CAD build for the part. Positions are in the model's coordinates, mm. A direction names the side the tool comes from. Give positions to 0.01 mm unless a question says otherwise; leave off trailing zeros. Loops run counter-clockwise (first coordinate to the right, second up) from the corner with the lowest first, then second, coordinate; pieces in that order, holes last. Notation, with made-up numbers: (25, 30) -> (59, 30) arc R15 ccw to (59, 42) -> close; hole circle Ø7 at (56, 12.5). An arc over 180 degrees is marked (long way). Write each question's results on one line, items separated by ' | '. Start each with the question number.
```python
from build123d import *

# Parameters (mm, degrees)
F0_R     = 50.8
F1_DEPTH = 10.16
F2_R     = 48.4632
F3_DEPTH = 10.16
F4_R     = 43.9928
F5_DEPTH = 10.16
F6_R     = 36.2712
F7_DEPTH = 10.16
F8_R     = 22.1488
F9_DEPTH = 10.16


with BuildPart() as f1:
    # F0 (on Top) → F1 (new body)
    with BuildSketch(Plane.XY):
        Circle(F0_R)
    extrude(amount=F1_DEPTH)

    # F2 (on face) → F3 (join)
    with BuildSketch(Plane.XY.offset(10.16)):
        Circle(F2_R)
    extrude(amount=F3_DEPTH)

    # F4 (on face) → F5 (join)
    with BuildSketch(Plane.XY.offset(20.32)):
        Circle(F4_R)
    extrude(amount=F5_DEPTH)

    # F6 (on face) → F7 (join)
    with BuildSketch(Plane.XY.offset(30.48)):
        Circle(F6_R)
    extrude(amount=F7_DEPTH)

    # F8 (on face) → F9 (join)
    with BuildSketch(Plane.XY.offset(40.64)):
        Circle(F8_R)
    extrude(amount=F9_DEPTH)


solid = f1.part
```
Q1. Which spindle directions (+Z, -Z, +X, -X, +Y, -Y) get a long thin tool onto all of the face, cutting with end or side? Do faces 1 (the face through (-34.91, -26.77, 25.33)), 2 (the face through (0, 0, 50.8)). Say none if no direction does.
Q2. Drop flat-ended pins along their axis: pin 1 (4 mm diameter, centred on x = -4.5, z = 10.5, fed in from -Y); pin 2 (4 mm diameter, centred on x = -20, y = 25.5, fed in from +Z); pin 3 (1 mm diameter, centred on y = -2, z = 13, fed in from +X). Give the stop position or say it passes through.
Q3. Saw through at A-A, the plane x = 0. List the corners of the cut face in (y, z), then the cut area to 3 significant figures.
Q4. Wall check: L1, parallel to Z at x = 2, y = 36; L2, parallel to Z at x = -22.5, y = -39; L3, parallel to X at y = 6, z = 4.5. Give the ranges that are in metal, low to high.
Q5. Saw through at D-D, the plane x = -25. List the corners of the cut face in (y, z), then the cut area to 3 significant figures.
Q6. Saw through at C-C, the plane z = 15. List the corners of the cut face in (x, y).
Answer block:
1) face 1: +Z | face 2: +Z, +X, -X, +Y, -Y
2) pin 1: stops at y = -50.74 | pin 2: stops at z = 40.64 | pin 3: stops at x = 48.44
3) outline: (-50.8, 0) -> (50.8, 0) -> (50.8, 10.16) -> (48.46, 10.16) -> (48.46, 20.32) -> (43.99, 20.32) -> (43.99, 30.48) -> (36.27, 30.48) -> (36.27, 40.64) -> (22.15, 40.64) -> (22.15, 50.8) -> (-22.15, 50.8) -> (-22.15, 40.64) -> (-36.27, 40.64) -> (-36.27, 30.48) -> (-43.99, 30.48) -> (-43.99, 20.32) -> (-48.46, 20.32) -> (-48.46, 10.16) -> (-50.8, 10.16) -> close | area: 4,100 mm2
4) L1: z = 0 to 40.64 | L2: z = 0 to 20.32 | L3: x = -50.44 to 50.44
5) outline: (-44.22, 0) -> (44.22, 0) -> (44.22, 10.16) -> (41.52, 10.16) -> (41.52, 20.32) -> (36.2, 20.32) -> (36.2, 30.48) -> (26.28, 30.48) -> (26.28, 40.64) -> (-26.28, 40.64) -> (-26.28, 30.48) -> (-36.2, 30.48) -> (-36.2, 20.32) -> (-41.52, 20.32) -> (-41.52, 10.16) -> (-44.22, 10.16) -> close | area: 3,010 mm2
6) outline: circle Ø96.93 at (0, 0)
